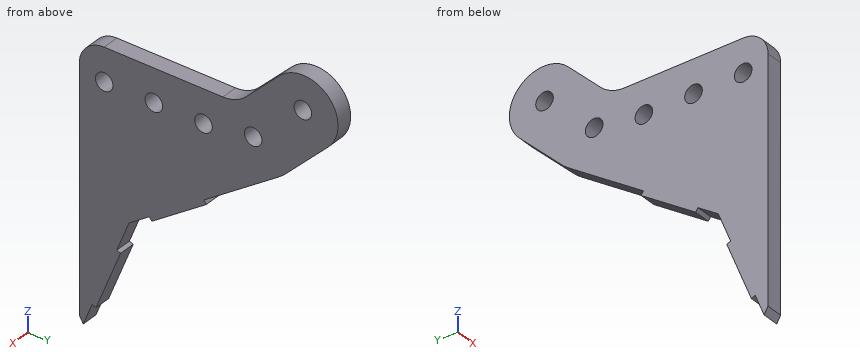
```python
from build123d import *

# Parameters (mm, degrees)
SKETCH1_R                   = 19.05
BOSS_EXTRUDE1_DEPTH         = 12.7
FILLET1_R                   = 25.4
FILLET2_R                   = 50.8
F_1_2_CLEARANCE_HOLE1_D     = 13.49248
F_1_2_CLEARANCE_HOLE1_DEPTH = 38.1
F_1_2_CLEARANCE_HOLE1_TIP   = 4.053549943
SKETCH4_R                   = 19.05
CUT_EXTRUDE1_DEPTH          = 13.7
BOSS_EXTRUDE2_DEPTH         = 12.7
BOSS_EXTRUDE3_DEPTH         = 12.7
FILLET3_R                   = 19.05
CHAMFER1_SIZE               = 12.7
CHAMFER1_SIZE2              = 8.080195177


with BuildPart() as part:
    # Sketch1 → Boss-Extrude1 (new body)
    with BuildSketch(Plane(origin=(0, 0, 0), x_dir=(0, 0, -1), z_dir=(1, 0, 0))):
        with BuildLine():
            Line((390.630407277, -109.766978243), (305.29908743, -24.435658396))
            Line((305.29908743, -24.435658396), (12.395871839, 49.264412727))
            ThreePointArc((12.395871839, 49.264412727), (-49.470959365, 11.544010545), (-10.688712274, -49.662777107))
            Line((-10.688712274, -49.662777107), (281.610658396, -75.235658396))
            Line((281.610658396, -75.235658396), (339.725, -133.35))
            Line((339.725, -133.35), (339.725, -254))
            Line((339.725, -254), (390.630407277, -254))
            Line((390.630407277, -254), (390.630407277, -109.766978243))
        make_face()
        Circle(SKETCH1_R, mode=Mode.SUBTRACT)
    extrude(amount=BOSS_EXTRUDE1_DEPTH)

    # Fillet1
    fillet1_edges = [part.edges().sort_by_distance(p)[0] for p in [
        (6.35, -133.35, -339.725),
        (6.35, -75.235658396, -281.610658396),
    ]]
    fillet(fillet1_edges, radius=FILLET1_R)

    # Fillet2
    fillet2_edges = [part.edges().sort_by_distance(p)[0] for p in [
        (6.35, -24.435658396, -305.29908743),
        (6.35, -109.766978243, -390.630407277),
    ]]
    fillet(fillet2_edges, radius=FILLET2_R)

    # 1/2 Clearance Hole1
    with Locations(Plane(origin=(12.7, 0, 0), x_dir=(0, 0, -1), z_dir=(1, 0, 0))):
        with Locations((365.125, -234.95), (365.125, -196.85), (365.125, -158.75), (359.5071206, -120.65), (324.846024484, -82.55)):
            Hole(F_1_2_CLEARANCE_HOLE1_D / 2, depth=F_1_2_CLEARANCE_HOLE1_DEPTH)
            with Locations((0, 0, -(F_1_2_CLEARANCE_HOLE1_DEPTH + F_1_2_CLEARANCE_HOLE1_TIP / 2))):  # 118° drill point
                Cone(0, F_1_2_CLEARANCE_HOLE1_D / 2, F_1_2_CLEARANCE_HOLE1_TIP, mode=Mode.SUBTRACT)

    # Sketch4 → Cut-Extrude1 (cut, through all)
    with BuildSketch(Plane(origin=(12.7, 0, 0), x_dir=(0, 0, -1), z_dir=(1, 0, 0))):
        with BuildLine():
            Line((288.147750244, -81.772750244), (306.885512242, -100.510512242))
            ThreePointArc((306.885512242, -100.510512242), (306.885512242, -63.266297725), (344.129726759, -63.266297725))
            Line((344.129726759, -63.266297725), (315.219181895, -34.355752861))
            ThreePointArc((315.219181895, -34.355752861), (304.360921026, -26.089699144), (291.69402925, -21.012364618))
            Line((291.69402925, -21.012364618), (12.395871839, 49.264412727))
            ThreePointArc((12.395871839, 49.264412727), (-49.470959365, 11.544010545), (-10.688712274, -49.662777107))
            Line((-10.688712274, -49.662777107), (272.400993868, -74.429917155))
            ThreePointArc((272.400993868, -74.429917155), (280.92174185, -76.713044696), (288.147750244, -81.772750244))
        make_face()
        Circle(SKETCH4_R, mode=Mode.SUBTRACT)
    extrude(amount=-CUT_EXTRUDE1_DEPTH, mode=Mode.SUBTRACT)

    # Sketch5 → Boss-Extrude2 (add)
    with BuildSketch(Plane(origin=(12.7, 0, 0), x_dir=(0, 0, -1), z_dir=(1, 0, 0))):
        with BuildLine():
            Line((390.630407277, -254), (555.730407277, -254))
            Line((555.730407277, -254), (460.480407277, -215.9))
            Line((460.480407277, -215.9), (381.605516519, -101.904352022))
            ThreePointArc((381.605516519, -101.904352022), (388.321723765, -115.668610267), (390.630407277, -130.809027211))
            Line((390.630407277, -130.809027211), (390.630407277, -254))
        make_face()
    extrude(amount=-BOSS_EXTRUDE2_DEPTH)

    # Sketch6 → Boss-Extrude3 (add)
    with BuildSketch(Plane(origin=(12.7, 0, 0), x_dir=(0, 0, -1), z_dir=(1, 0, 0))):
        Polygon((449.641154081, -200.234334034), (452.252098409, -198.427791835), (423.347423219, -156.652682593), (420.736478891, -158.459224792), align=None)
        Polygon((484.063715226, -225.333323179), (485.242880623, -222.385409686), (532.40949652, -241.252056045), (531.230331123, -244.199969538), align=None)
    extrude(amount=-BOSS_EXTRUDE3_DEPTH)

    # Fillet3
    fillet3_edges = [part.edges().sort_by_distance(p)[0] for p in [
        (6.35, -254, -339.725),
    ]]
    fillet(fillet3_edges, radius=FILLET3_R)

    # Chamfer1
    chamfer1_edges = [part.edges().sort_by_distance(p)[0] for p in [
        (6.35, -254, -555.730407277),
    ]]
    chamfer1_side = [part.faces().sort_by_distance(p)[0] for p in [
        (6.35, -254, -457.252703639),
    ]]
    chamfer(chamfer1_edges, length=CHAMFER1_SIZE, length2=CHAMFER1_SIZE2, reference=chamfer1_side[0])


solid = part.part
```
CAD build for the part. Positions are in the model's coordinates, mm. Coordinates: 2 decimals unless noted, no trailing zeros. Write each loop counter-clockwise with the first axis right and the second up, starting at its lowest first coordinate (ties: lowest second). Pieces come first, ordered by that corner, then holes.
(1) Cut at C-C, the plane y = -120.65. List the corners of the cut face in (x, z) (3 decimals).
(2) Cut at A-A, the plane y = -82.55. List the corners of the cut face in (x, z), and give its area (3 significant figures).
(3) Cut at B-B, the plane x = 10.5. Count the separate pieces of the cut face and the enclosed holes in it, and give its area (3 significant figures).
(4) Drill centre lines: probe 1 along Z at (x, y) = (7, -126.5); probe 2 along Z at (x, y) = (3.25, -201) (3 decimals); probe 3 along Y at (x, z) = (11.5, -388). Where is each one in solid material? Low to high.
(5) Flat gauge pins, fed straight in: pin 1 (4 mm diameter, centred on x = 4, y = -174.5, fed in from +Z) (3 decimals); pin 2 (3 mm diameter, centred on x = 5.5, y = -126.5, fed in from +Z) (3 decimals); pin 3 (5 mm diameter, centred on x = 8, z = -356, fed in from -Y). Where does each tip first touch, or does it go through?
(6) Cut at D-D, the plane z = -396. List the corners of the cut face in (x, y).
Geometry says:
1. outline: (0, -394.576) - (12.7, -394.576) - (12.7, -366.253) - (0, -366.253) - close; (0, -352.761) - (12.7, -352.761) - (12.7, -327.025) - (0, -327.025) - close
2. outline: (0, -363.41) - (12.7, -363.41) - (12.7, -331.59) - (0, -331.59) - close; (0, -318.1) - (12.7, -318.1) - (12.7, -299.18) - (0, -299.18) - close
2. area: 644 mm2
3. separate pieces: 1
3. enclosed holes: 5
3. area: 18,300 mm2
4. probe 1: z = -398.62 to -362.87, -356.15 to -332.86
4. probe 2: z = -450.171 to -370.444, -359.806 to -339.725
4. probe 3: y = -254 to -111.15
5. pin 1: stops at z = -339.725
5. pin 2: stops at z = -331.375
5. pin 3: stops at y = -254
6. outline: (0, -254) - (12.7, -254) - (12.7, -122.71) - (0, -122.71) - close
